Design review of the part built by this model. Coordinates are the model's own, in mm. A direction names the side the tool comes from. Coordinates: 2 decimals unless noted, no trailing zeros. Write each loop counter-clockwise with the first axis right and the second up, starting at its lowest first coordinate (ties: lowest second). Pieces come first, ordered by that corner, then holes. Notation, with made-up numbers: (-17.5, -24) -> (-13.5, -24) arc R37 cw to (-13.5, 15) -> close; hole circle Ø5 at (21.5, -21.75). An arc over 180 degrees is marked (long way). One line per question, with ' | ' between items. Start each with the question number.
Q1. Wall thickness on probe 1 along Y at (x, z) = (10.5, 21); probe 2 along Z at (x, y) = (0, 84.5); probe 3 along Z at (x, y) = (20, 2): over which ranges is each line inside the solid? List them lowest first.
Q2. Add section A-A on x = -20. State the section outline as (y, z) points, and give its area (3 significant figures).
Q3. For P1, Ø3, axis at x = -8.5, y = 122.5, coming from the +Z side; P2, Ø8, axis at y = 36.5, z = -13.5, coming from the -X side; P3, Ø6, axis at y = 96, z = 8, coming from the -X side; P4, Ø5, axis at y = 89, z = -2, coming from the +X side, all flat-tipped, find the tip position at first contact; note any pin that passes through.
Q4. Add section C-C on x = 20.25. State the section outline as (y, z) points, and give its area (3 significant figures).
Q5. Add section D-D on z = 21. State the section outline as (x, y) points, and give its area (3 significant figures).
Q6. For faces 5 (the flat face through (-4.684, 91.13, -8.266)), 6 (the flat face through (4.8, 32.9, -8.2)), 7 (the conical face through (-0.02, 29.21, -9.86)), list the 3-axis set-ups (+Z, -Z, +X, -X, +Y, -Y) from which the entire face can be reached by the end or side of a thin tool; tool diameter is ignored.
Q7. Add section B-B on y = 27. State the section outline as (x, z) points, and give its area (3 significant figures).
Q8. Draft analysis for pull direction X (two halves, no side actions). For faces 1 (the cylindrical face through (5.723, 61.256, -1.802)), 2 (the flat face through (0, 137, 0)), 3 (the flat face through (-4.8, 91.1, 8.2)), 4 (the cylindrical face through (-17, 3, 0)), state which applies: pulls with the +X half, pulls with the -X half, needs draft (parallel to the pull), parting line crosses it, or undercut.
from build123d import *

# Parameters (mm, degrees)
EXTRUDE_1_DEPTH     = 8
EXTRUDE_2_DEPTH     = 10
SKETCH_5_R          = 3.25
CUT_EXTRUDE_1_DEPTH = 7


with BuildPart() as part:
    # Эскиз1 → Повернуть1 (revolve)
    with BuildSketch(Plane.XY, mode=Mode.PRIVATE) as revolve_1_sk:
        Polygon((0, 0), (-25, 0), (-25, 6), (-15, 6), (-11, 20), (-9, 20), (-9, 22), (-6, 25), (-6, 29), (-6, 37), (-6, 135.4), (-4.4, 137), (0, 137), align=None)
    revolve(revolve_1_sk.sketch.rotate(Axis((0, 0, 0), (0, 1, 0)), 180), axis=Axis((0, 0, 0), (0, 1, 0)))  # turned: the seam where the file's is

    # Эскиз2 → Бобышка-Вытянуть1 (add)
    with BuildSketch(Plane(origin=(0, 29, 0), x_dir=(1, 0, 0), z_dir=(0, 1, 0))):
        Polygon((0, 10.969655115), (-9.5, 5.484827557), (-9.5, -5.484827557), (0, -10.969655115), (9.5, -5.484827557), (9.5, 5.484827557), align=None)
    extrude(amount=EXTRUDE_1_DEPTH)

    # Эскиз3 → Бобышка-Вытянуть2 (add)
    with BuildSketch(Plane(origin=(0, 86.2, 0), x_dir=(1, 0, 0), z_dir=(0, 1, 0))):
        Polygon((9.5, 5.484827557), (0, 10.969655115), (-9.5, 5.484827557), (-9.5, -5.484827557), (0, -10.969655115), (9.5, -5.484827557), align=None)
    extrude(amount=EXTRUDE_2_DEPTH)

    # Эскиз4 → Вырез-Повернуть2 (revolve, cut)
    with BuildSketch(Plane.XY, mode=Mode.PRIVATE) as cut_revolve_2_sk:
        Polygon((-18.160254038, 96.2), (-9.5, 96.2), (-18.160254038, 91.2), align=None)
        Polygon((-18.160254038, 86.2), (-18.160254038, 91.2), (-9.5, 86.2), align=None)
        Polygon((-16.42820323, 37), (-16.42820323, 33), (-9.5, 37), align=None)
        Polygon((-16.42820323, 33), (-16.42820323, 29), (-9.5, 29), align=None)
    revolve(cut_revolve_2_sk.sketch.rotate(Axis((0, 137, 0), (0, -1, 0)), 180), axis=Axis((0, 137, 0), (0, -1, 0)), mode=Mode.SUBTRACT)  # turned: the seam where the file's is

    # Эскиз5 → Вырез-Вытянуть1 (cut, through all)
    with BuildSketch(Plane(origin=(0, 6, 0), x_dir=(1, 0, 0), z_dir=(0, 1, 0))):
        with Locations(Location((-20.25, 0, 0), (0, 0, 180))):  # turned: the seam where the file's is
            Circle(SKETCH_5_R)
        with Locations(Location((20.25, 0, 0), (0, 0, 180))):  # turned: the seam where the file's is
            Circle(SKETCH_5_R)
    extrude(amount=-CUT_EXTRUDE_1_DEPTH, mode=Mode.SUBTRACT)


solid = part.part
Output values:
1) probe 1: y = 0 to 6 | probe 2: z = -6 to 6 | probe 3: z = -15 to -3.24, 3.24 to 15
2) outline: (0, -15) -> (6, -15) -> (6, -3.24) -> (0, -3.24) -> close; (0, 3.24) -> (6, 3.24) -> (6, 15) -> (0, 15) -> close | area: 141 mm2
3) P1: passes through | P2: stops at x = -2.55 | P3: stops at x = -9.5 | P4: stops at x = 9.5
4) outline: (0, -14.66) -> (6, -14.66) -> (6, -3.25) -> (0, -3.25) -> close; (0, 3.25) -> (6, 3.25) -> (6, 14.66) -> (0, 14.66) -> close | area: 137 mm2
5) outline: (-13.56, 0) -> (13.56, 0) -> (13.56, 6) -> (-13.56, 6) -> close | area: 163 mm2
6) face 5: -Z, -X, +Y | face 6: -Z, +X, +Y | face 7: -Z
7) outline: circle Ø12 at (0, 0) | area: 113 mm2
8) face 1: parting line crosses it | face 2: needs draft | face 3: pulls with the -X half | face 4: undercut
